Input: part model. Units: mm. Frame: model coordinates. Face numbers are marked on the shaded views. A direction names the side the tool comes from. Coordinates: 2 decimals unless noted, no trailing zeros. Loops run counter-clockwise (first coordinate to the right, second up) from the corner with the lowest first, then second, coordinate; pieces in that order, holes last.
Item 1: Pull-direction query (X, two-part tool) for the marked faces 5, 6 and 7; classes: released by +X, released by -X, zero draft, split by the parting line, or undercut.
Item 2: Section A-A on y = 13.5. Return loops of the section in (x, z), and give its area (3 significant figures).
Item 3: Ray query, line 1 along Y through (x, z) = (0, -5.2); line 2 along Y through (x, z) = (-7.5, -1.5); line 3 along Y through (x, z) = (-7.25, 0). Return the intervals inside material, ascending.
Item 4: Contact query for flat-ended pins moving along their axis: P1, Ø3, axis at x = 0, y = -9.48, coming from the +Z side; P2, Ø2, axis at y = -9.48, z = 0, coming from the +X side; P3, Ø2.5, axis at x = 0.5, y = -9, coming from the -Z side; P4, Ø6.5, axis at x = 0, z = 0, coming from the -Y side. Output: stop coordinate, or through.
Item 5: Reachability of the marked faces 1, 2, 3 and 4 from +Z, -Z, +X, -X, +Y, -Y: full face, straight path, thin tool, end or side. Return the list, or none.
Autodesk Inventor part; units mm, degrees
ref_plane "YZ Plane" through (0, 0, 0) normal (1, 0, 0) x (0, 1, 0)
ref_plane "XZ Plane" through (0, 0, 0) normal (0, 1, 0) x (-1, 0, 0)
ref_plane "XY Plane" through (0, 0, 0) normal (0, 0, 1) x (1, 0, 0)
sketch "Sketch1" plane through (0, 0, 0) normal (0, 0, 1) x (1, 0, 0)
  line L0 (0, 0) -> (8.4519, 0)
  line L1 (8.4519, 0) -> (8.4519, 12.7)
  line L2 (8.4519, 12.7) -> (7.0041, 12.7)
  line L3 (7.0041, 12.7) -> (7.0041, 15.113)
  line L4 (7.0041, 15.113) -> (8.4519, 15.113)
  line L5 (8.4519, 15.113) -> (8.4519, 18.288)
  line L6 (8.4519, 18.288) -> (0, 18.288)
  line L7 (0, 18.288) -> (0, 0)
  line L8 (0, -29.2334) -> (0, 26.2082)
  line L9 (8.4519, 0) -> (8.4519, 6.35)
  line L10 (8.4519, 0) -> (8.4519, 6.35)
  line L11 (8.4519, 6.35) -> (15.4293, -8.6131)
  line L12 (8.4519, 6.35) -> (24.9619, 6.35) construction
  line L13 (15.4293, -8.6131) -> (12.2543, -8.6131)
  line L14 (12.2543, -8.6131) -> (8.4519, 0)
  line L15 (15.4293, -8.6131) -> (0, -8.6131)
  line L16 (0, 0) -> (8.4519, 0)
  line L17 (0, -8.6131) -> (12.7, -8.6131)
  line L18 (12.7, -8.6131) -> (12.7, -21.3131)
  line L19 (12.7, -21.3131) -> (0, -21.3131)
  line L20 (0, -21.3131) -> (0, -8.6131)
  line L21 (12.7, -8.6131) -> (12.7, -2.7602)
  point P0 (12.2543, -8.6131)
  dimension "d0" = 8.4519
  dimension "d1" = 12.7
  dimension "d2" = 90
  dimension "d3" = 1.4478
  dimension "d4" = 2.413
  dimension "d5" = 3.175
  dimension "d23" = 16.51
  dimension "d24" = 65
  dimension "d25" = 3.175
  dimension "d83" = 12.7
  dimension "d84" = 12.7
revolve "Revolution1" add sketch "Sketch1" angle 360 about axis through (0, -10, 0) along (0, 1, 0) contours L7 L6 L5 L4 L3 L2 L1 L0 | L0 L14 L15 L8 | L1 L11 L21 L13 L14 | L15 L13 L18 L19 L8
sketch "Sketch12" plane through (0, 18.288, 0) normal (0, 1, 0) x (1, 0, 0)
  point P0 (0, 0)
  point P1 (0, 0)
hole "Hole4" at (0, 18.288, 0) direction (0, -1, 0) diameter 1.5875 depth 32.8676 tip angle 118
sketch "Sketch13" plane through (0, -21.3131, 0) normal (0, -1, 0) x (1, 0, 0)
  circle A0 centre (0, 0) radius 12.7
  point P0 (12.7, 0)
  point P1 (0, -12.7)
  point P2 (-12.7, 0)
  point P3 (0, 12.7)
ref_plane "Work Plane1" through (12.7, -21.3131, 0) normal (1, 0, 0) x (0, 1, 0)
sketch "Sketch14" plane through (12.7, -21.3131, 0) normal (1, 0, 0) x (0, 1, 0)
  line L0 (0, 12.7) -> (0, -12.7)
  line L1 (0, 0) -> (18.553, 0)
  line L2 (18.553, 12.7) -> (18.553, -12.7)
  line L3 (18.553, 0) -> (11.8347, 0)
  point P0 (21.3131, 0)
  dimension "d92" = 6.7183
hole "Hole5" at (12.7, -9.4785, 0) direction (-1, 0, 0) diameter 1.5875 end through all
hole "Hole6" at (12.7, -9.4785, 0) direction (-1, 0, 0) diameter 5.3594 depth 6.35
extrude "Extrusion3" add sketch "Sketch13" along normal blind 6.35
sketch "Sketch16" plane through (0, -27.6631, 0) normal (0, -1, 0) x (1, 0, 0)
  point P0 (0, 0)
hole "Hole8" at (0, -27.6631, 0) direction (0, 1, 0) diameter 4.9784 depth 6.35
pattern_circular "Circular Pattern5" count 4 over 360 about axis through (0, -10, 0) along (0, 1, 0) of "Hole5", "Hole6"
equation "\"d54\" = 55deg"
equation "\"Sketch7_Pitch\" = 0.90714"
equation "\"d72\" = 55deg"
equation "\"Sketch9_Pitch\" = 1.27"
equation "\"d137\" = 55deg"
equation "\"Sketch17_Pitch\" = 1.27"
equation "\"d155\" = 55deg"
equation "\"Sketch19_Pitch\" = 0.90714"
equation "\"d173\" = 55deg"
equation "\"Sketch21_Pitch\" = 0.90714"
equation "\"d191\" = 55deg"
equation "\"Sketch23_Pitch\" = 1.27"
equation "\"d221\" = 55deg"
equation "\"Sketch25_Pitch\" = 0.90714"
equation "\"d239\" = 55deg"
equation "\"Sketch27_Pitch\" = 1.27"
properties part number "piston badflowchannel-1-16in-thread"
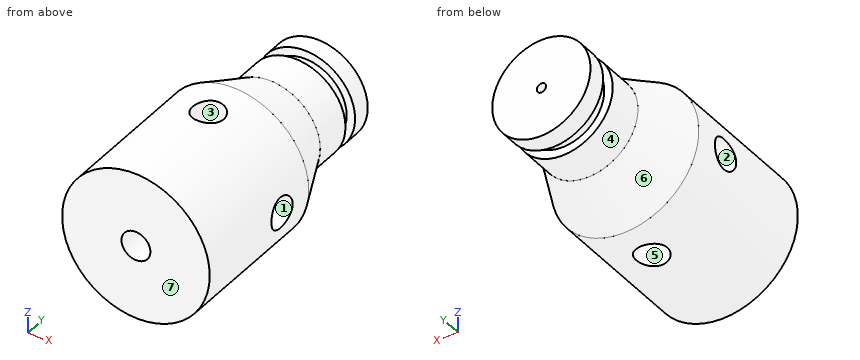
Results found:
1. face 5: undercut
1. face 6: split by the parting line
1. face 7: zero draft
2. outline: circle Ø14.01 at (0, 0); hole circle Ø1.59 at (0, 0)
2. area: 152 mm2
3. line 1: y = -27.66 to -10.27, -8.68 to 18.29
3. line 2: y = -27.66 to -11.7, -7.26 to 12.7, 15.11 to 18.29
3. line 3: y = -27.66 to -12.16, -6.8 to 12.7, 15.11 to 18.29
4. P1: stops at z = 6.35
4. P2: stops at x = 6.35
4. P3: stops at z = -6.35
4. P4: stops at y = -27.66
5. face 1: +X
5. face 2: -X
5. face 3: +Z
5. face 4: +Y
